Build history of the part. All positions in model axes, mm. Face numbers are marked on the shaded views. A direction names the side the tool comes from. Round coordinates to 2 decimals unless told otherwise and drop trailing zeros. Write each loop counter-clockwise with the first axis right and the second up, starting at its lowest first coordinate (ties: lowest second). Pieces come first, ordered by that corner, then holes. Notation, with made-up numbers: (3, 10.5) -> (40, 10.5) arc R6 ccw to (40, 18.5) -> close; hole circle Ø1 at (-4, -21.75). An arc over 180 degrees is marked (long way). One line per question, with ' | ' between items.
from build123d import *

# Parameters (mm, degrees)
PAD_DEPTH    = 10
SKETCH001_W  = 2.5
SKETCH001_H  = 10
PAD001_DEPTH = 8
SKETCH002_R  = 1.5
POCKET_DEPTH = 2.501
FILLET_R     = 4


with BuildPart() as part:
    # Sketch → Pad (new body)
    with BuildSketch(Plane.XY):
        with BuildLine():
            ThreePointArc((10.5, 12.5), (11.277816, 8.461126), (13.5, 5))
            Line((13.5, 5), (27.5, 5))
            ThreePointArc((27.5, 5), (29.722184, 8.461126), (30.5, 12.5))
            Line((33, 12.5), (30.5, 12.5))
            Line((33, 2.5), (33, 12.5))
            Line((8, 2.5), (33, 2.5))
            Line((8, 10), (8, 2.5))
            Line((0, 10), (8, 10))
            Line((0, 12.5), (0, 10))
            Line((8, 12.5), (0, 12.5))
            Line((10.5, 12.5), (8, 12.5))
        make_face()
    extrude(amount=PAD_DEPTH)

    # Sketch001 (on Face5 of Pad) → Pad001 (join)
    with BuildSketch(Plane.YZ.offset(33)):
        with Locations((11.25, 5)):
            Rectangle(SKETCH001_W, SKETCH001_H)
    extrude(amount=PAD001_DEPTH)

    # Sketch002 (on Face10 of Pad001) → Pocket (cut, through all)
    with BuildSketch(Plane.XZ.offset(-10)):
        with Locations((4, 5)):
            Circle(SKETCH002_R)
        with Locations((37, 5)):
            Circle(SKETCH002_R)
    extrude(amount=-POCKET_DEPTH, mode=Mode.SUBTRACT)

    # Fillet
    fillet_edges = [part.edges().sort_by_distance(p)[0] for p in [
        (8, 2.5, 5),
        (33, 2.5, 5),
    ]]
    fillet(fillet_edges, radius=FILLET_R)


solid = part.part
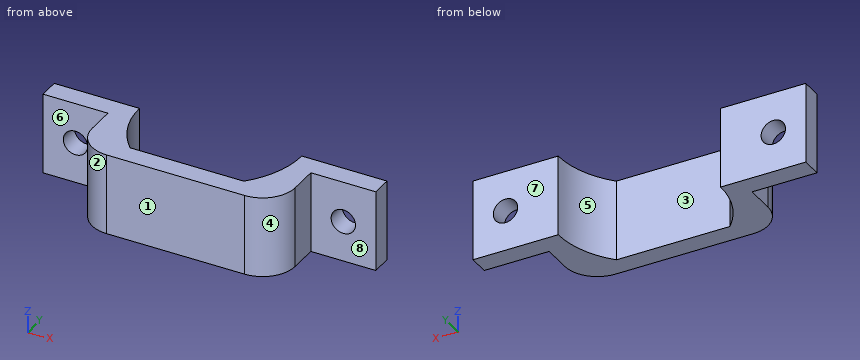
(1) Wall check: line 1 (Z direction, x = 37, y = 11); line 2 (X direction, y = 7, z = 1.75); line 3 (X direction, y = 6, z = 7.5). Give the ranges that are in metal, low to high. Write a range as from..to.
Calculated:
line 1: 0..3.5, 6.5..10 | line 2: 8..11.99, 29.01..33 | line 3: 8.03..12.66, 28.34..32.97
(2) Mould opens along X. For the marked faces 1, 2, 3 and 4 say: pulls with the +X half, pulls with the -X half, needs draft (parallel to the pull), parting line crosses it, or undercut.
Calculated:
face 1: needs draft | face 2: pulls with the -X half | face 3: undercut | face 4: pulls with the +X half
(3) Slice it at B-B (x = 37). Write the cut outline in (y, z), then the cut area to 3 significant figures.
Calculated:
outline: (10, 0) -> (12.5, 0) -> (12.5, 3.5) -> (10, 3.5) -> close; (10, 6.5) -> (12.5, 6.5) -> (12.5, 10) -> (10, 10) -> close | area: 17.5 mm2
(4) Drop flat-ended pins along their axis: pin 1 (3 mm diameter, centred on x = 6, y = 4.5, fed in from +Z); pin 2 (4 mm diameter, centred on x = 7, z = 4.5, fed in from -Y); pin 3 (4 mm diameter, centred on x = 3, z = 6.5, fed in from -Y); pin 4 (4 mm diameter, centred on y = 7.5, z = 7, fed in from -X). Give the stop position or say it passes through.
Calculated:
pin 1: through | pin 2: y = 3.85 | pin 3: y = 10 | pin 4: x = 8
(5) Slice it at C-C (y = 5.5). Write the cut outline in (x, z), then the cut area to 3 significant figures.
Calculated:
outline: (8.13, 0) -> (13.05, 0) -> (13.05, 10) -> (8.13, 10) -> close; (27.95, 0) -> (32.87, 0) -> (32.87, 10) -> (27.95, 10) -> close | area: 98.5 mm2
(6) Slice it at D-D (z = 1.75). Write the cut outline in (x, y) (3 decimals).
Calculated:
outline: (0, 10) -> (8, 10) -> (8, 6.5) arc R4 ccw to (12, 2.5) -> (29, 2.5) arc R4 ccw to (33, 6.5) -> (33, 10) -> (41, 10) -> (41, 12.5) -> (30.5, 12.5) arc R10.875 cw to (27.5, 5) -> (13.5, 5) arc R10.875 cw to (10.5, 12.5) -> (0, 12.5) -> close
(7) Slice it at A-A (z = 5). Write the cut outline in (x, y) (3 decimals), then the cut area to 3 significant figures.
Calculated:
outline: (0, 10) -> (2.5, 10) -> (2.5, 12.5) -> (0, 12.5) -> close; (5.5, 10) -> (8, 10) -> (8, 6.5) arc R4 ccw to (12, 2.5) -> (29, 2.5) arc R4 ccw to (33, 6.5) -> (33, 10) -> (35.5, 10) -> (35.5, 12.5) -> (30.5, 12.5) arc R10.875 cw to (27.5, 5) -> (13.5, 5) arc R10.875 cw to (10.5, 12.5) -> (5.5, 12.5) -> close; (38.5, 10) -> (41, 10) -> (41, 12.5) -> (38.5, 12.5) -> close | area: 132 mm2
(8) 3-axis set-ups, long thin cutter, end or side, ignore diameter. For the marked faces 5, 6, 7 and 8: which of +Z, -Z, +X, -X, +Y, -Y reach the whole face in a straight line?
Calculated:
face 5: +Z, -Z, +Y | face 6: +Z, -Z, -X, -Y | face 7: +Z, -Z, +X, -X, +Y | face 8: +Z, -Z, +X, -Y
